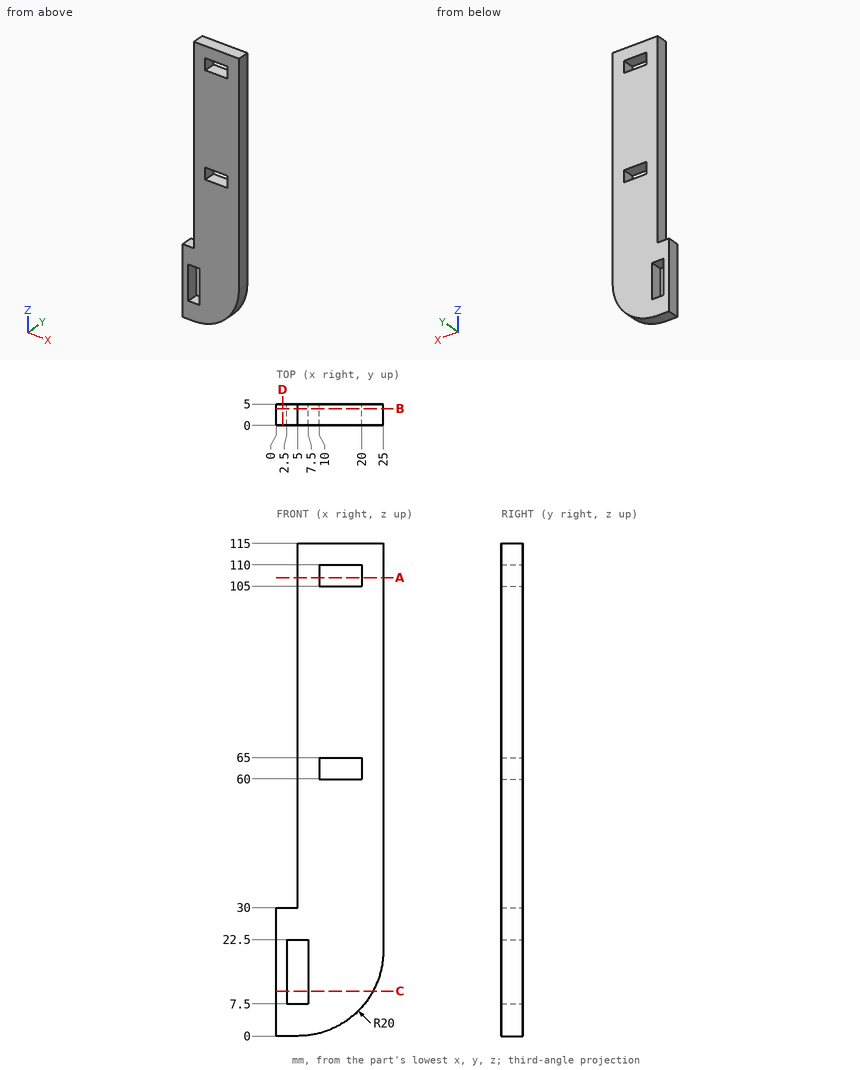
Geometry: see drawing. Coordinates: mm, zero at the bounding-box minimum. Round coordinates to 2 decimals unless told otherwise and drop trailing zeros. Write each loop counter-clockwise with the first axis right and the second up, starting at its lowest first coordinate (ties: lowest second). Pieces come first, ordered by that corner, then holes.
Item 1: Section query D-D (x = 1.5). Return loops of the section in (y, z).
Item 2: Section query B-B (y = 3.9). Return loops of the section in (x, z), plus the area to 3 significant figures.
Item 3: Pin query (flat end, axial travel): P1, Ø2.5, axis at y = 2, z = 63, coming from the -X side; P2, Ø1.5, axis at x = 2, y = 2, coming from the +Z side; P3, Ø1.5, axis at x = 17.5, y = 1, coming from the -Z side. Return the tip coordinate at first contact, or that it passes through.
Item 4: Section query C-C (z = 10.5). Return loops of the section in (x, y).
Item 5: Section query A-A (z = 107). Return loops of the section in (x, y), plus the area to 3 significant figures.
Item 6: Material intervals for L1, parallel to Z at x = 12.5, y = 4.5; L2, parallel to Z at x = 12, y = 4.15 (3 decimals); L3, parallel to Z at x = 3, y = 4, sorted ascending.
Completed:
1. outline: (0, 0) - (5, 0) - (5, 30) - (0, 30) - close
2. outline: (0, 0) - (5, 0) arc R20 ccw to (25, 20) - (25, 115) - (5, 115) - (5, 30) - (0, 30) - close; hole (2.5, 7.5) - (7.5, 7.5) - (7.5, 22.5) - (2.5, 22.5) - close; hole (10, 60) - (20, 60) - (20, 65) - (10, 65) - close; hole (10, 105) - (20, 105) - (20, 110) - (10, 110) - close
2. area: 2,190 mm2
3. P1: stops at x = 5
3. P2: stops at z = 30
3. P3: stops at z = 3.82
4. outline: (0, 0) - (2.5, 0) - (2.5, 5) - (0, 5) - close; (7.5, 0) - (22.6, 0) - (22.6, 5) - (7.5, 5) - close
5. outline: (5, 0) - (10, 0) - (10, 5) - (5, 5) - close; (20, 0) - (25, 0) - (25, 5) - (20, 5) - close
5. area: 50.0 mm2
6. L1: z = 1.46 to 60, 65 to 105, 110 to 115
6. L2: z = 1.265 to 60, 65 to 105, 110 to 115
6. L3: z = 0 to 7.5, 22.5 to 30
